Geometry check sheet. Reference: the model listing, model coordinates, mm. Face numbers are marked on the shaded views. A direction names the side the tool comes from. Give positions to 0.01 mm unless a question says otherwise; leave off trailing zeros. Order: outer loops, then holes, each group sorted by start corner. A loop starts at its lowest first (then second) coordinate and runs counter-clockwise, first axis right, second up. Notation, with made-up numbers: M 75,-21 L 92,-21 A22 cw 92,13 Z; hole C -4,65.5 d1. An arc over 180 degrees is marked long. Answer as CSV lines item,"result". Start each with the question number.
Q1. Mould release check, pull along Y, two halves, no side actions. Record for the marked faces 1, 2 and 3: +Y half, -Y half, draft (parallel to the pull), parting line (faces both ways), or undercut.
Q2. Set-up check for the marked faces 4 and 5: record each of +Z, -Z, +X, -X, +Y, -Y from which the full face is reachable in a straight line by a thin tool's end or side.
Q3. Section check C-C, the plane z = -1.5. Record the boundary of the cut face in (x, y) (3 decimals).
Q4. Go/stop test with flat-tipped pins: pin 1 (5 mm diameter, centred on x = -1, y = -1.5, fed in from -Z); pin 2 (2 mm diameter, centred on x = -1.5, z = -2.5, fed in from +Y). Record where each tip stops, or that it passes through.
Q5. Thickness scan on line 1 (Y direction, x = 0, z = -1.95) (3 decimals); line 2 (X direction, y = -0.25, z = -0.65); line 3 (Y direction, x = 2.5, z = -0.85). Record the ranges inside material, lowest first.
Q6. Section check A-A, the plane x = 0. Record the boundary of the cut face in (y, z) (3 decimals).
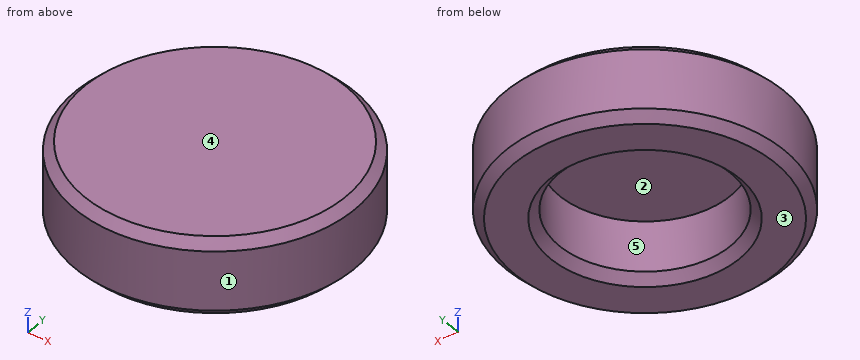
Autodesk Fusion 360 part; units mm, degrees
sketch "Sketch1" plane through (0, 0, 0) normal (0, 0, 1) x (1, 0, 0)
  circle A0 centre (0, 0) radius 7.775
  circle A1 centre (0, 0) radius 4.775
  dimension "d1" = 9.55
  dimension "d2" = 15.55
extrude "Extrude1" add sketch "Sketch1" along normal blind 1 contours A0 | A1
extrude "Extrude2" add sketch "Sketch1" against normal blind 3.3
chamfer "Chamfer1" distance 0.5 angle 45 3 edges at (-7.2488, -2.8116, 1) (-7.2488, 2.8116, -3.3) (-4.4519, -1.7267, -3.3)
equation "d2 = d1 + 6 mm"
Answer block:
1,face 1,"parting line"
1,face 2,"undercut"
1,face 3,"draft"
2,face 4,"+Z, +X, -X, +Y, -Y"
2,face 5,"-Z"
3,outline,"C 0,0 d15.55; hole C 0,0 d9.55"
4,pin 1,"stops at z = 0"
4,pin 2,"stops at y = 7.76"
5,line 1,"y = -7.775 to -4.775, 4.775 to 7.775"
5,line 2,"x = -7.77 to -4.77, 4.77 to 7.77"
5,line 3,"y = -7.36 to -4.07, 4.07 to 7.36"
6,outline,"M -7.775,-2.8 L -7.275,-3.3 L -5.275,-3.3 L -4.775,-2.8 L -4.775,0 L 4.775,0 L 4.775,-2.8 L 5.275,-3.3 L 7.275,-3.3 L 7.775,-2.8 L 7.775,0.5 L 7.275,1 L -7.275,1 L -7.775,0.5 Z"
